Source: CAD feature listing. Evaluate the final solid. Frame: model axes, mm. Face numbers are marked on the shaded views. A direction names the side the tool comes from. Round coordinates to 2 decimals unless told otherwise and drop trailing zeros. Order: outer loops, then holes, each group sorted by start corner. A loop starts at its lowest first (then second) coordinate and runs counter-clockwise, first axis right, second up. Notation, with made-up numbers: M 52,-10 L 95,-10 A23 ccw 95,20 Z; hole C -27,89.5 d7. An arc over 180 degrees is marked long. Answer in a Markdown table with one row per item. Add a question column.
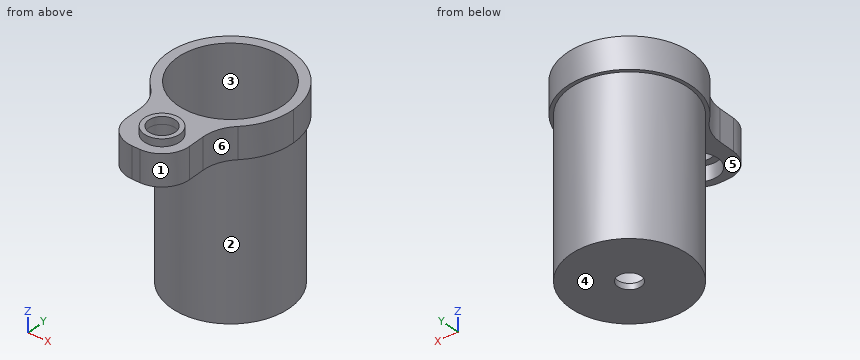
```python
from build123d import *

# Parameters (mm, degrees)
F1_DEPTH  = 8
F2_R      = 15.1
F3_DEPTH  = 40
F4_R      = 7
F5_R      = 13.5
F6_DEPTH  = 46.5
F7_R      = 4.55
F7_R_2    = 3.4
F8_DEPTH  = 1.9
F9_DEPTH  = 48.001
F10_R     = 5.125
F10_R_2   = 3.4
F11_DEPTH = 3.75
F12_R     = 3
F13_DEPTH = 49.901
F14_R     = 10


with BuildPart() as f1:
    # F0 (on Top) → F1 (new body)
    with BuildSketch(Plane.XY):
        with BuildLine():
            ThreePointArc((8, -13.8564064606), (13.8564064606, -8), (16, 0))
            ThreePointArc((16, 0), (-8, 13.8564064606), (-8, -13.8564064606))
            Line((-8, -13.8564064606), (-8, 0))
            Line((-8, 0), (8, 0))
            Line((8, 0), (8, -13.8564064606))
        make_face()
        with BuildLine():
            Line((-8, 0), (-8, -13.8564064606))
            ThreePointArc((-8, -13.8564064606), (0, -16), (8, -13.8564064606))
            Line((8, -13.8564064606), (8, 0))
            Line((8, 0), (-8, 0))
        make_face()
        with BuildLine():
            ThreePointArc((8, -13.8564064606), (0, -16), (-8, -13.8564064606))
            Line((-8, -13.8564064606), (-8, -30))
            Line((-8, -30), (8, -30))
            Line((8, -30), (8, -13.8564064606))
        make_face()
    extrude(amount=F1_DEPTH)

    # F2 (on face) → F3 (join)
    with BuildSketch(Plane(origin=(0, 0, 0), x_dir=(1, 0, 0), z_dir=(0, 0, -1))):
        Circle(F2_R)
    extrude(amount=F3_DEPTH)

    # F4
    f4_edges = [f1.edges().sort_by_distance(p)[0] for p in [
        (-8, -30, 4),
        (8, -30, 4),
    ]]
    fillet(f4_edges, radius=F4_R)

    # F5 (on face) → F6 (cut)
    with BuildSketch(Plane.XY.offset(8)):
        Circle(F5_R)
    extrude(amount=-F6_DEPTH, mode=Mode.SUBTRACT)

    # F7 (on face) → F8 (join)
    with BuildSketch(Plane.XY.offset(8)):
        with Locations((1, -23)):
            Circle(F7_R)
        with Locations((1, -23)):
            Circle(F7_R_2, mode=Mode.SUBTRACT)
    extrude(amount=F8_DEPTH)

    # F9 (cut, through all): a face of the model
    f9_faces = [f1.faces().sort_by_distance(p)[0] for p in [
        (1, -23, 8),
    ]]
    extrude(f9_faces, amount=-F9_DEPTH, mode=Mode.SUBTRACT)

    # F10 (on face) → F11 (cut)
    with BuildSketch(Plane(origin=(0, 0, 0), x_dir=(1, 0, 0), z_dir=(0, 0, -1))):
        with Locations((1, 23)):
            Circle(F10_R)
        with Locations((1, 23)):
            Circle(F10_R_2, mode=Mode.SUBTRACT)
    extrude(amount=-F11_DEPTH, mode=Mode.SUBTRACT)

    # F12 (on face) → F13 (cut, through all)
    with BuildSketch(Plane(origin=(0, 0, -40), x_dir=(1, 0, 0), z_dir=(0, 0, -1))):
        Circle(F12_R)
    extrude(amount=-F13_DEPTH, mode=Mode.SUBTRACT)

    # F14
    f14_edges = [f1.edges().sort_by_distance(p)[0] for p in [
        (-8, -13.856406, 4),
        (8, -13.856406, 4),
    ]]
    fillet(f14_edges, radius=F14_R)


solid = f1.part
```
(1) Cut plane B-B (y = -25.5). Return loops of the section in (x, z).
(2) Draft query along Y for the marked faces 1, 2, 3 and 4. Return one class per face: +Y half, -Y half, draft (parallel to the pull), parting line (faces both ways), or undercut.
(3) Line query: line 1 (X direction, y = -23, z = 1.4) (3 decimals); line 2 (X direction, y = 0, z = -39.3); line 3 (Y direction, x = 1, z = 9). Output: solid intervals per line, ascending. Write a range as from..to.
(4) Access query for the marked faces 5 and 6. Directions: +Z, -Z, +X, -X, +Y, -Y. A direction counts if a zero-diameter tool reaches every point of the face in a straight line with its end or side. Return the directions, or none.
(5) Cut plane A-A (z = 3). Return loops of the section in (x, y) (3 decimals).
(6) Cut plane D-D (y = 1.5). Return loops of the section in (x, z).
(7) Cut plane C-C (x = 0). Return loops of the section in (y, z).
(8) Pin query (flat end, axial travel): pin 1 (2 mm diameter, centred on y = -20, z = 3, fed in from +X); pin 2 (10 mm diameter, centred on x = 12, y = -18.5, fed in from +Z); pin 3 (5 mm diameter, centred on y = -4, z = -15.5, fed in from +X). Return the tip coordinate at first contact, or that it passes through.
Answer list:
| question | item | result |
|---|---|---|
| 1 | outline | M -7.54,0 L -3.47,0 L -3.47,3.75 L -1.3,3.75 L -1.3,9.9 L -2.8,9.9 L -2.8,8 L -7.54,8 Z; M 3.3,3.75 L 5.47,3.75 L 5.47,0 L 7.54,0 L 7.54,8 L 4.8,8 L 4.8,9.9 L 3.3,9.9 Z |
| 2 | face 1 | -Y half |
| 2 | face 2 | parting line |
| 2 | face 3 | undercut |
| 2 | face 4 | draft |
| 3 | line 1 | -8..-4.125, 6.125..8 |
| 3 | line 2 | -15.1..-3, 3..15.1 |
| 3 | line 3 | -27.55..-26.4, -19.6..-18.45 |
| 4 | face 5 | -Z |
| 4 | face 6 | +Z, -Z, +X, -Y |
| 5 | outline | M -11.077,-11.546 A10 cw -8,-18.762 L -8,-23 A7 ccw -1,-30 L 1,-30 A7 ccw 8,-23 L 8,-18.762 A10 cw 11.077,-11.546 A16 ccw long Z; hole C 0,0 d27; hole C 1,-23 d10.25 |
| 6 | outline | M -15.93,0 L -15.03,0 L -15.03,-40 L -2.6,-40 L -2.6,-38.5 L -13.42,-38.5 L -13.42,8 L -15.93,8 Z; M 2.6,-40 L 15.03,-40 L 15.03,0 L 15.93,0 L 15.93,8 L 13.42,8 L 13.42,-38.5 L 2.6,-38.5 Z |
| 7 | outline | M -30,0 L -28.03,0 L -28.03,3.75 L -26.25,3.75 L -26.25,9.9 L -27.44,9.9 L -27.44,8 L -30,8 Z; M -19.75,3.75 L -17.97,3.75 L -17.97,0 L -15.1,0 L -15.1,-40 L -3,-40 L -3,-38.5 L -13.5,-38.5 L -13.5,8 L -18.56,8 L -18.56,9.9 L -19.75,9.9 Z; M 3,-40 L 15.1,-40 L 15.1,0 L 16,0 L 16,8 L 13.5,8 L 13.5,-38.5 L 3,-38.5 Z |
| 8 | pin 1 | x = 8 |
| 8 | pin 2 | z = 8 |
| 8 | pin 3 | x = 15.03 |
